For this review, take the finished solid that the model builds, in its own axes (mm). A direction names the side the tool comes from. Round coordinates to 2 decimals unless told otherwise and drop trailing zeros. Order: outer loops, then holes, each group sorted by start corner. A loop starts at its lowest first (then second) coordinate and runs counter-clockwise, first axis right, second up. Notation, with made-up numbers: M 72,-27.5 L 76,-27.5 A19 cw 76,-1.5 Z; hole C 74.5,-7.5 d3. An arc over 180 degrees is marked long. Put each result on its own line as item: value.
from build123d import *

# Parameters (mm, degrees)
SKETCH1_R           = 2.5
SKETCH1_W           = 40
SKETCH1_H           = 6.35
BOSS_EXTRUDE1_DEPTH = 6.35
SKETCH2_R           = 3.2
CUT_EXTRUDE1_DEPTH  = 6.35


with BuildPart() as part:
    # Sketch1 → Boss-Extrude1 (new body)
    with BuildSketch(Plane(origin=(0, 0, 0), x_dir=(1, 0, 0), z_dir=(0, 1, 0))):
        with BuildLine():
            ThreePointArc((171.132486541, -50), (181.122528791, -25.88190451), (184.529946162, 0))
            ThreePointArc((184.529946162, 0), (181.122528791, 25.88190451), (171.132486541, 50))
            Line((171.132486541, 50), (128.867513459, 123.205080757))
            ThreePointArc((128.867513459, 123.205080757), (92.264973081, 159.807621135), (42.264973081, 173.205080757))
            Line((42.264973081, 173.205080757), (-42.264973081, 173.205080757))
            ThreePointArc((-42.264973081, 173.205080757), (-92.264973081, 159.807621135), (-128.867513459, 123.205080757))
            Line((-128.867513459, 123.205080757), (-171.132486541, 50))
            ThreePointArc((-171.132486541, 50), (-184.529946162, 0), (-171.132486541, -50))
            Line((-171.132486541, -50), (-128.867513459, -123.205080757))
            ThreePointArc((-128.867513459, -123.205080757), (-92.264973081, -159.807621135), (-42.264973081, -173.205080757))
            Line((-42.264973081, -173.205080757), (42.264973081, -173.205080757))
            ThreePointArc((42.264973081, -173.205080757), (92.264973081, -159.807621135), (128.867513459, -123.205080757))
            Line((128.867513459, -123.205080757), (171.132486541, -50))
        make_face()
        with Locations(Location((-92.611215932, -143.407331345, 0), (0, 0, 270))):
            Circle(SKETCH1_R, mode=Mode.SUBTRACT)
        with Locations(Location((-77.888784068, -151.907331345, 0), (0, 0, 270))):
            Circle(SKETCH1_R, mode=Mode.SUBTRACT)
        Polygon((-38.958176102, -92.977540378), (-35.927087189, -94.727540378), (-42.427087189, -105.985870628), (-62.427087189, -140.626886779), (-68.927087189, -151.885217028), (-71.958176102, -150.135217028), (-94.041823898, -137.385217028), (-97.072912811, -135.635217028), (-90.572912811, -124.376886779), (-70.572912811, -89.735870628), (-64.072912811, -78.477540378), (-61.041823898, -80.227540378), align=None, mode=Mode.SUBTRACT)
        with Locations(Location((-40.388784068, -86.955426061, 0), (0, 0, 270))):
            Circle(SKETCH1_R, mode=Mode.SUBTRACT)
        Polygon((-145.403071882, -60.854491924), (-139.903810568, -57.679491924), (-119.903810568, -92.320508076), (-125.403071882, -95.495508076), align=None, mode=Mode.SUBTRACT)
        with Locations(Location((-170.5, -8.5, 0), (0, 0, 270))):
            Circle(SKETCH1_R, mode=Mode.SUBTRACT)
        Polygon((-100, -12.75), (-100, -16.25), (-113, -16.25), (-153, -16.25), (-166, -16.25), (-166, -12.75), (-166, 12.75), (-166, 16.25), (-153, 16.25), (-113, 16.25), (-100, 16.25), (-100, 12.75), align=None, mode=Mode.SUBTRACT)
        with Locations(Location((-95.5, -8.5, 0), (0, 0, 270))):
            Circle(SKETCH1_R, mode=Mode.SUBTRACT)
        with Locations(Location((-55.111215932, -78.455426061, 0), (0, 0, 270))):
            Circle(SKETCH1_R, mode=Mode.SUBTRACT)
        with Locations((0, -153.175)):
            Rectangle(SKETCH1_W, SKETCH1_H, mode=Mode.SUBTRACT)
        with Locations(Location((77.888784068, -151.907331345, 0), (0, 0, 270))):
            Circle(SKETCH1_R, mode=Mode.SUBTRACT)
        with Locations(Location((40.388784068, -86.955426061, 0), (0, 0, 270))):
            Circle(SKETCH1_R, mode=Mode.SUBTRACT)
        Polygon((61.041823898, -80.227540378), (64.072912811, -78.477540378), (70.572912811, -89.735870628), (90.572912811, -124.376886779), (97.072912811, -135.635217028), (94.041823898, -137.385217028), (71.958176102, -150.135217028), (68.927087189, -151.885217028), (62.427087189, -140.626886779), (42.427087189, -105.985870628), (35.927087189, -94.727540378), (38.958176102, -92.977540378), align=None, mode=Mode.SUBTRACT)
        with Locations(Location((92.611215932, -143.407331345, 0), (0, 0, 270))):
            Circle(SKETCH1_R, mode=Mode.SUBTRACT)
        with Locations(Location((55.111215932, -78.455426061, 0), (0, 0, 270))):
            Circle(SKETCH1_R, mode=Mode.SUBTRACT)
        Polygon((125.403071882, -95.495508076), (119.903810568, -92.320508076), (139.903810568, -57.679491924), (145.403071882, -60.854491924), align=None, mode=Mode.SUBTRACT)
        with Locations(Location((95.5, -8.5, 0), (0, 0, 270))):
            Circle(SKETCH1_R, mode=Mode.SUBTRACT)
        with Locations(Location((170.5, -8.5, 0), (0, 0, 270))):
            Circle(SKETCH1_R, mode=Mode.SUBTRACT)
        with Locations(Location((-170.5, 8.5, 0), (0, 0, 270))):
            Circle(SKETCH1_R, mode=Mode.SUBTRACT)
        with Locations(Location((-95.5, 8.5, 0), (0, 0, 270))):
            Circle(SKETCH1_R, mode=Mode.SUBTRACT)
        Polygon((-125.403071882, 95.495508076), (-119.903810568, 92.320508076), (-139.903810568, 57.679491924), (-145.403071882, 60.854491924), align=None, mode=Mode.SUBTRACT)
        with Locations(Location((-55.111215932, 78.455426061, 0), (0, 0, 270))):
            Circle(SKETCH1_R, mode=Mode.SUBTRACT)
        with Locations(Location((-92.611215932, 143.407331345, 0), (0, 0, 270))):
            Circle(SKETCH1_R, mode=Mode.SUBTRACT)
        Polygon((-61.041823898, 80.227540378), (-64.072912811, 78.477540378), (-70.572912811, 89.735870628), (-90.572912811, 124.376886779), (-97.072912811, 135.635217028), (-94.041823898, 137.385217028), (-71.958176102, 150.135217028), (-68.927087189, 151.885217028), (-62.427087189, 140.626886779), (-42.427087189, 105.985870628), (-35.927087189, 94.727540378), (-38.958176102, 92.977540378), align=None, mode=Mode.SUBTRACT)
        with Locations(Location((-40.388784068, 86.955426061, 0), (0, 0, 270))):
            Circle(SKETCH1_R, mode=Mode.SUBTRACT)
        with Locations(Location((-77.888784068, 151.907331345, 0), (0, 0, 270))):
            Circle(SKETCH1_R, mode=Mode.SUBTRACT)
        with Locations(Location((55.111215932, 78.455426061, 0), (0, 0, 270))):
            Circle(SKETCH1_R, mode=Mode.SUBTRACT)
        with Locations(Location((95.5, 8.5, 0), (0, 0, 270))):
            Circle(SKETCH1_R, mode=Mode.SUBTRACT)
        Polygon((100, -12.75), (100, 0), (100, 12.75), (100, 16.25), (113, 16.25), (153, 16.25), (166, 16.25), (166, 12.75), (166, 0), (166, -12.75), (166, -16.25), (153, -16.25), (113, -16.25), (100, -16.25), align=None, mode=Mode.SUBTRACT)
        with Locations(Location((170.5, 8.5, 0), (0, 0, 270))):
            Circle(SKETCH1_R, mode=Mode.SUBTRACT)
        Polygon((145.403071882, 60.854491924), (139.903810568, 57.679491924), (119.903810568, 92.320508076), (125.403071882, 95.495508076), align=None, mode=Mode.SUBTRACT)
        with Locations(Location((40.388784068, 86.955426061, 0), (0, 0, 270))):
            Circle(SKETCH1_R, mode=Mode.SUBTRACT)
        Polygon((38.958176102, 92.977540378), (35.927087189, 94.727540378), (42.427087189, 105.985870628), (62.427087189, 140.626886779), (68.927087189, 151.885217028), (71.958176102, 150.135217028), (94.041823898, 137.385217028), (97.072912811, 135.635217028), (90.572912811, 124.376886779), (70.572912811, 89.735870628), (64.072912811, 78.477540378), (61.041823898, 80.227540378), align=None, mode=Mode.SUBTRACT)
        with Locations((0, 153.175)):
            Rectangle(SKETCH1_W, SKETCH1_H, mode=Mode.SUBTRACT)
        with Locations(Location((77.888784068, 151.907331345, 0), (0, 0, 270))):
            Circle(SKETCH1_R, mode=Mode.SUBTRACT)
        with Locations(Location((92.611215932, 143.407331345, 0), (0, 0, 270))):
            Circle(SKETCH1_R, mode=Mode.SUBTRACT)
    extrude(amount=BOSS_EXTRUDE1_DEPTH)

    # Sketch2 → Cut-Extrude1 (cut)
    with BuildSketch(Plane(origin=(0, 6.35, 0), x_dir=(1, 0, 0), z_dir=(0, 1, 0))):
        with Locations(Location((55.794244464, -33.346698257, 0), (0, 0, 270))):
            Circle(SKETCH2_R)
        with Locations(Location((-56.776210055, -31.645883963, 0), (0, 0, 270))):
            Circle(SKETCH2_R)
        with Locations(Location((0.981965591, 64.99258222, 0), (0, 0, 270))):
            Circle(SKETCH2_R)
    extrude(amount=-CUT_EXTRUDE1_DEPTH, mode=Mode.SUBTRACT)


solid = part.part
(1) For faces 1 (the face through (-150.296, 3.131, 86.09)), 2 (the face through (-130.044, 3.131, 74.758)), list the 3-axis set-ups (+Z, -Z, +X, -X, +Y, -Y) from which the entire face can be reached by the end or side of a thin tool; tool diameter is ignored.
A:
face 1: +Z, -X, +Y, -Y
face 2: +Y, -Y
(2) Add section B-B on z = 130. Give the boundary of the cut face in (x, y).
A:
outline: M -124.57,0 L -93.82,0 L -93.82,6.35 L -124.57,6.35 Z; M -56.29,0 L 56.29,0 L 56.29,6.35 L -56.29,6.35 Z; M 93.82,0 L 124.57,0 L 124.57,6.35 L 93.82,6.35 Z
(3) To check wall thickness, follow L1, parallel to Z at x = 10, y = 4; L2, parallel to Z at x = -38.5, y = 4.5; L3, parallel to Z at x = -122.5, y = 5.25. State the ranges of each line that lie inside material, in increasing order.
A:
L1: z = -173.21 to -156.35, -150 to 150, 156.35 to 173.21
L2: z = -173.21 to -99.18, -93.24 to -88.59, -85.32 to 85.32, 88.59 to 93.24, 99.18 to 173.21
L3: z = -132.89 to -93.82, -87.82 to -16.25, 16.25 to 87.82, 93.82 to 132.89
(4) Insertion check: pin 1 Ø1 at (y, z) = (3, 21) entering from -X; pin 2 Ø4 at (x, z) = (-56.78, 31.65) entering from +Y; pin 3 Ø2 at (y, z) = (3.5, -107.5) entering from +X; pin 4 Ø1.5 at (y, z) = (4.5, -59) entering from +X. Each pin has a flat end and moves straight along its axis. Give the tip position at first contact, or say it passes through.
A:
pin 1: stops at x = -182.41
pin 2: passes through
pin 3: stops at x = 138.51
pin 4: stops at x = 166.37
(5) Add section A-A on x = -158. Give the boundary of the cut face in (y, z).
A:
outline: M 0,-72.75 L 6.35,-72.75 L 6.35,-16.25 L 0,-16.25 Z; M 0,16.25 L 6.35,16.25 L 6.35,72.75 L 0,72.75 Z
(6) Add section D-D on z = 43. Give the boundary of the cut face in (x, y), then the cut area to 3 significant figures.
A:
outline: M -174.81,0 L 174.81,0 L 174.81,6.35 L -174.81,6.35 Z
area: 2,220 mm2
(7) Draft analysis for pull direction Z (two halves, no side actions). For faces 3 (the face through (-3, 0, -2)), 4 (the face through (-135.26, 3.13, 78.42)), 5 (the face through (92.9, 3.13, -159.44)), state which applies: released by +Z, released by -Z, zero draft, split by the parting line, or undercut.
A:
face 3: zero draft
face 4: undercut
face 5: released by -Z
(8) Add section C-C on y = 5. State how many separate pieces and enclosed holes the cut face has, then the cut area to 3 significant figures.
A:
separate pieces: 1
enclosed holes: 39
area: 85,700 mm2
